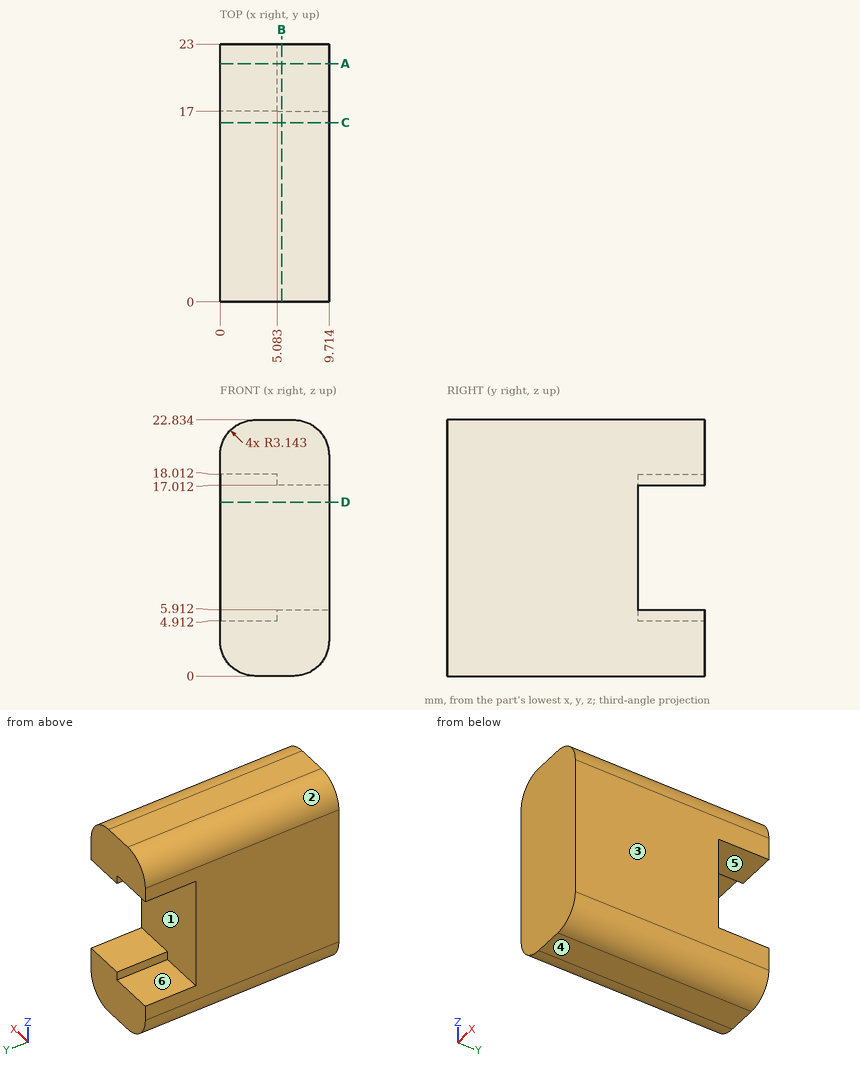
Source: three-view drawing plus pictorial views. Frame: mm from the lowest corner of the part. A direction names the side the tool comes from. Round coordinates to 2 decimals unless told otherwise and drop trailing zeros. Loops run counter-clockwise (first coordinate to the right, second up) from the corner with the lowest first, then second, coordinate; pieces in that order, holes last. Notation, with made-up numbers: (14.25, 57.5) - (38.25, 57.5) arc R10 ccw to (38.25, 67.5) - close; hole circle Ø6 at (43, -13.75). An arc over 180 degrees is marked (long way). Write each question's results on one line, items separated by ' | '. Start each with the question number.
1) Mould query, pull axis Z, two halves, no side actions, for the marked faces 1, 2 and 3. Classes: released by +Z, released by -Z, zero draft, split by the parting line, or undercut.
2) Cut plane B-B on x = 5.5. Return loops of the section in (y, z).
3) First-contact query: P1, Ø2.5, axis at x = 1.5, y = 21, coming from the -Z side (1 decimal); P2, Ø3, axis at x = 1.5, y = 16, coming from the +Z side; P3, Ø3, axis at y = 20, z = 6.5, coming from the -X side. Flat tips, straight axial feed; report the tip coordinate or a pass-through.
4) Cut plane A-A on y = 21.25. Return loops of the section in (x, z) (1 decimal).
5) Access query for the marked faces 4, 5 and 6. Directions: +Z, -Z, +X, -X, +Y, -Y. A direction counts if a zero-diameter tool reaches every point of the face in a straight line with its end or side. Return the directions, or none.
6) Line query: probe 1 along Z at (x, y) = (3.25, 19); probe 2 along Z at (x, y) = (6, 19.5); probe 3 along Y at (x, z) = (8.5, 6.25). Output: solid intervals per line, ascending. Write a range as [from, to].
7) Cut plane D-D on z = 15.5. Return loops of the section in (x, y) (1 decimal).
8) Cut plane C-C on y = 16. Return loops of the section in (x, z) (1 decimal), then the cut area to 3 significant figures.
Verdict:
1) face 1: undercut | face 2: released by +Z | face 3: zero draft
2) outline: (0, 0) - (23, 0) - (23, 5.91) - (17, 5.91) - (17, 17.01) - (23, 17.01) - (23, 22.83) - (0, 22.83) - close
3) P1: stops at z = 0 | P2: stops at z = 22.83 | P3: stops at x = 5.08
4) outline: (0, 3.1) arc R3.1 ccw to (3.1, 0) - (6.6, 0) arc R3.1 ccw to (9.7, 3.1) - (9.7, 5.9) - (5.1, 5.9) - (5.1, 4.9) - (0, 4.9) - close; (0, 18) - (5.1, 18) - (5.1, 17) - (9.7, 17) - (9.7, 19.7) arc R3.1 ccw to (6.6, 22.8) - (3.1, 22.8) arc R3.1 ccw to (0, 19.7) - close
5) face 4: -Z, +X, -X, +Y, -Y | face 5: +X, -X, +Y | face 6: -X, +Y
6) probe 1: z = [0, 4.91], [18.01, 22.83] | probe 2: z = [0, 5.91], [17.01, 22.83] | probe 3: y = [0, 17]
7) outline: (0, 0) - (9.7, 0) - (9.7, 17) - (0, 17) - close
8) outline: (0, 3.1) arc R3.1 ccw to (3.1, 0) - (6.6, 0) arc R3.1 ccw to (9.7, 3.1) - (9.7, 19.7) arc R3.1 ccw to (6.6, 22.8) - (3.1, 22.8) arc R3.1 ccw to (0, 19.7) - close | area: 213 mm2
